Build history of the part. All positions in model axes, mm. Face numbers are marked on the shaded views. A direction names the side the tool comes from. Give positions to 0.01 mm unless a question says otherwise; leave off trailing zeros. Order: outer loops, then holes, each group sorted by start corner. A loop starts at its lowest first (then second) coordinate and runs counter-clockwise, first axis right, second up. Notation, with made-up numbers: M 40.5,-15.5 L 77.5,-15.5 A28 ccw 77.5,20.5 Z; hole C 23,84.25 d5. An arc over 180 degrees is marked long. Answer as CSV lines item,"result".
from build123d import *

# Parameters (mm, degrees)
F1_DEPTH = 50
F2_W     = 100
F2_H     = 120
F3_DEPTH = 2
F5_D     = 10
F6_W     = 79.999998
F6_H     = 100.000001
F7_DEPTH = 2


with BuildPart() as f1:
    # F0 (on Front) → F1 (new body, symmetric)
    with BuildSketch(Plane.XZ):
        Polygon((50, -60), (50, 0), (50, 60), (-50, 60), (-50, -60), align=None)
        Polygon((-48, -58), (-48, 58), (48, 58), (48, 0), (48, -58), align=None, mode=Mode.SUBTRACT)
    extrude(amount=F1_DEPTH, both=True)

    # F2 (on face) → F3 (join)
    with BuildSketch(Plane(origin=(0, 50, 0), x_dir=(-1, 0, 0), z_dir=(0, 1, 0))):
        Rectangle(F2_W, F2_H)
    extrude(amount=-F3_DEPTH)

    # F5 (through all)
    with Locations(Plane(origin=(0, 50, 0), x_dir=(-1, 0, 0), z_dir=(0, 1, 0))):
        with Locations((0, 0)):
            Hole(F5_D / 2)

    # F6 (on face) → F7 (join)
    with BuildSketch(Plane.XZ.offset(50)):
        Polygon((50, 55), (50, 60), (-50, 60), (-50, -60), (50, -60), align=None)
        with Locations((0, 0)):
            Rectangle(F6_W, F6_H, mode=Mode.SUBTRACT)
    extrude(amount=-F7_DEPTH)


solid = f1.part
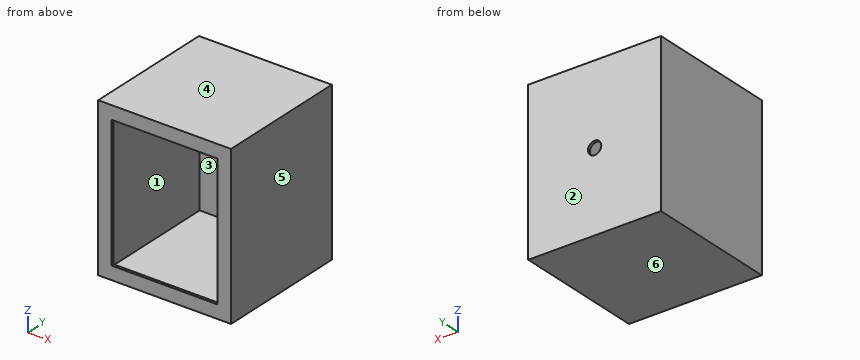
Item 1: Band-saw the part on C-C (z = 0). Give the cut face in (x, y), and give its area (3 significant figures).
Geometry says:
outline,"M -50,-50 L -40,-50 L -40,-48 L -48,-48 L -48,48 L -5,48 L -5,50 L -50,50 Z; M 5,48 L 48,48 L 48,-48 L 40,-48 L 40,-50 L 50,-50 L 50,50 L 5,50 Z"
area,"604 mm2"
Item 2: Band-saw the part on B-B (x = 0). Give the cut face in (y, z).
Geometry says:
outline,"M -50,-60 L 50,-60 L 50,-5 L 48,-5 L 48,-58 L -48,-58 L -48,-50 L -50,-50 Z; M -50,50 L -48,50 L -48,58 L 48,58 L 48,5 L 50,5 L 50,60 L -50,60 Z"
Item 3: Probe line 1 along X through (y, z) = (-2.5, 37); line 2 along Z through (x, y) = (0, 49.15). List the from-to ranges inside material, lowest first. Write a range as from..to.
Geometry says:
line 1,"x = -50..-48, 48..50"
line 2,"z = -60..-5, 5..60"
Item 4: 3-axis set-ups, long thin cutter, end or side, ignore diameter. For the marked faces 1 and 2: which of +Z, -Z, +X, -X, +Y, -Y reach the whole face in a straight line?
Geometry says:
face 1,"none"
face 2,"+Z, -Z, +X, -X, +Y"
Item 5: Pull direction Z, two halves, no side cores. Call the marked faces 3, 4, 5 and 6: released by +Z, released by -Z, zero draft, split by the parting line, or undercut.
Geometry says:
face 3,"undercut"
face 4,"released by +Z"
face 5,"zero draft"
face 6,"released by -Z"
Item 6: Band-saw the part on A-A (z = -52). Give the cut face in (x, y).
Geometry says:
outline,"M -50,-50 L 50,-50 L 50,50 L -50,50 Z; hole M -48,-48 L 48,-48 L 48,48 L -48,48 Z"
Item 7: Band-saw the part on D-D (y = 13). Give the cut face in (x, z).
Geometry says:
outline,"M -50,-60 L 50,-60 L 50,60 L -50,60 Z; hole M -48,-58 L 48,-58 L 48,58 L -48,58 Z"
Item 8: Drop a flat-ended pin along its axis: pin 1 (4 mm diameter, centred on x = -2.5, z = -17.5, fed in from -Y). Give the stop position or say it passes through.
Geometry says:
pin 1,"stops at y = 48"
